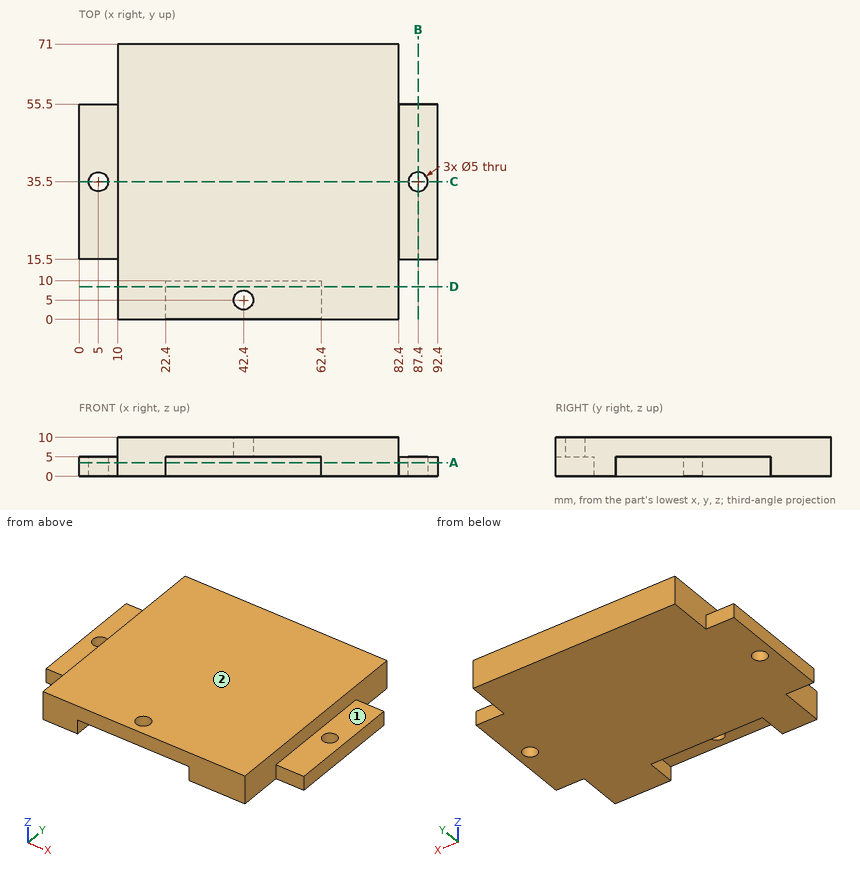
Input: dimensioned drawing with shaded views. Units: mm. Origin: part minimum x, y, z. A direction names the side the tool comes from. Coordinates: 2 decimals unless noted, no trailing zeros. Loops run counter-clockwise (first coordinate to the right, second up) from the corner with the lowest first, then second, coordinate; pieces in that order, holes last. Notation, with made-up numbers: M -20,-27 L -11,-27 A32 ccw -11,8 Z; hole C -38,43 d9. An arc over 180 degrees is marked long. Use a Markdown table: item, result. Add a question column.
Q1. Access query for the marked faces 1 and 2. Directions: +Z, -Z, +X, -X, +Y, -Y. A direction counts if a zero-diameter tool reaches every point of the face in a straight line with its end or side. Return the directions, or none.
Q2. Material intervals for L1, parallel to Y at x = 42.4, z = 8; L2, parallel to Y at x = 87.4, z = 1; L3, parallel to X at y = 37, z = 4.75, sorted ascending.
Q3. Section query A-A, the plane z = 3.5. Return loops of the section in (x, y).
Q4. Section query C-C, the plane y = 35.5. Return loops of the section in (x, z), and give its area (3 significant figures).
Q5. Section query D-D, the plane y = 8.5. Return loops of the section in (x, z), and give its area (3 significant figures).
Q6. First-contact query: pin 1 (2.5 mm diameter, centred on x = 88.5, z = 2.5, fed in from -Y); pin 2 (11 mm diameter, centred on x = 6.5, y = 43, fed in from +Z); pin 3 (1.5 mm diameter, centred on y = 62.5, z = 7, fed in from +X); pin 4 (5.5 mm diameter, centred on x = 89.5, z = 2, fed in from +Y). Flat tips, straight axial feed; report the tip coordinate or a pass-through.
Q7. Section query B-B, the plane x = 87.4. Return loops of the section in (y, z).
Result:
| question | item | result |
|---|---|---|
| 1 | face 1 | +Z, +X, +Y, -Y |
| 1 | face 2 | +Z, +X, -X, +Y, -Y |
| 2 | L1 | y = 0 to 2.5, 7.5 to 71 |
| 2 | L2 | y = 15.5 to 33, 38 to 55.5 |
| 2 | L3 | x = 0 to 3, 7 to 85.4, 89.4 to 92.4 |
| 3 | outline | M 0,15.5 L 10,15.5 L 10,0 L 22.4,0 L 22.4,10 L 62.4,10 L 62.4,0 L 82.4,0 L 82.4,15.5 L 92.4,15.5 L 92.4,55.5 L 82.4,55.5 L 82.4,71 L 10,71 L 10,55.5 L 0,55.5 Z; hole C 5,35.5 d5; hole C 87.4,35.5 d5 |
| 4 | outline | M 0,0 L 2.5,0 L 2.5,5 L 0,5 Z; M 7.5,0 L 84.9,0 L 84.9,5 L 82.4,5 L 82.4,10 L 10,10 L 10,5 L 7.5,5 Z; M 89.9,0 L 92.4,0 L 92.4,5 L 89.9,5 Z |
| 4 | area | 774 mm2 |
| 5 | outline | M 10,0 L 22.4,0 L 22.4,5 L 62.4,5 L 62.4,0 L 82.4,0 L 82.4,10 L 10,10 Z |
| 5 | area | 524 mm2 |
| 6 | pin 1 | stops at y = 15.5 |
| 6 | pin 2 | stops at z = 10 |
| 6 | pin 3 | stops at x = 82.4 |
| 6 | pin 4 | stops at y = 55.5 |
| 7 | outline | M 15.5,0 L 33,0 L 33,5 L 15.5,5 Z; M 38,0 L 55.5,0 L 55.5,5 L 38,5 Z |
